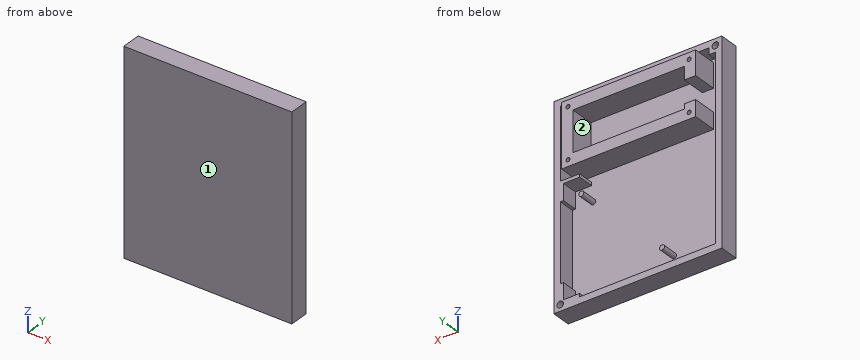
```python
from build123d import *

# Parameters (mm, degrees)
SKETCH1_W           = 104
SKETCH1_H           = 124
BOSS_EXTRUDE1_DEPTH = 2
SKETCH2_W           = 104
SKETCH2_H           = 124
SKETCH2_R           = 2
SKETCH2_R_2         = 1.55
BOSS_EXTRUDE2_DEPTH = 10
SKETCH3_R           = 1.25
BOSS_EXTRUDE3_DEPTH = 15


with BuildPart() as part:
    # Sketch1 → Boss-Extrude1 (new body)
    with BuildSketch(Plane(origin=(0, 0, 0), x_dir=(1, 0, 0), z_dir=(0, 1, 0))):
        Rectangle(SKETCH1_W, SKETCH1_H)
    extrude(amount=BOSS_EXTRUDE1_DEPTH)

    # Sketch2 → Boss-Extrude2 (add)
    # profile 1 of 3: a face of its own
    with BuildSketch(Plane(origin=(0, 2, 0), x_dir=(1, 0, 0), z_dir=(0, 1, 0))):
        Rectangle(SKETCH2_W, SKETCH2_H)
        Polygon((36, -14), (48, -14), (48, -58), (-44, -58), (-44, -54), (-48, -54), (-48, 58), (36, 58), (36, 56), (46, 56), (46, 46), (48, 46), (48, -2), (46, -2), (46, -12), (36, -12), align=None, mode=Mode.SUBTRACT)
        with Locations(Location((48, 58, 0), (0, 0, 270))):
            Circle(SKETCH2_R, mode=Mode.SUBTRACT)
        with Locations(Location((-48, -58, 0), (0, 0, 270))):
            Circle(SKETCH2_R, mode=Mode.SUBTRACT)
    # profile 2 of 3: a face of its own
    with BuildSketch(Plane(origin=(0, 2, 0), x_dir=(1, 0, 0), z_dir=(0, 1, 0))):
        with Locations(Location((-15, 48, 0), (0, 0, 90))):
            Circle(SKETCH2_R_2)
    # profile 3 of 3: a face of its own
    with BuildSketch(Plane(origin=(0, 2, 0), x_dir=(1, 0, 0), z_dir=(0, 1, 0))):
        with Locations(Location((35, -2, 0), (0, 0, 90))):
            Circle(SKETCH2_R_2)
    extrude(amount=BOSS_EXTRUDE2_DEPTH)

    # Sketch3 → Boss-Extrude3 (add)
    with BuildSketch(Plane(origin=(0, 2, 0), x_dir=(1, 0, 0), z_dir=(0, 1, 0))):
        Polygon((36.5, -49), (-32.5, -49), (-32.5, -41), (-39.5, -41), (-39.5, -56), (43.5, -56), (43.5, -17), (-39.5, -17), (-39.5, -27), (-32.5, -27), (-32.5, -24), (36.5, -24), align=None)
        with Locations(Location((-35.5, -52, 0), (0, 0, 270))):
            Circle(SKETCH3_R, mode=Mode.SUBTRACT)
        with Locations(Location((39.5, -52, 0), (0, 0, 270))):
            Circle(SKETCH3_R, mode=Mode.SUBTRACT)
        with Locations(Location((-35.5, -21, 0), (0, 0, 270))):
            Circle(SKETCH3_R, mode=Mode.SUBTRACT)
        with Locations(Location((39.5, -21, 0), (0, 0, 270))):
            Circle(SKETCH3_R, mode=Mode.SUBTRACT)
    extrude(amount=BOSS_EXTRUDE3_DEPTH)


solid = part.part
```
Can you work these out from the model? Positions are in its coordinate system, mm. Face numbers are marked on the shaded views. Round coordinates to 2 decimals unless told otherwise and drop trailing zeros. Loops run counter-clockwise (first coordinate to the right, second up) from the corner with the lowest first, then second, coordinate; pieces in that order, holes last.
Item 1: Suppose I cut it at B-B, the plane x = -24. Write out the boundary of the cut face in (y, z), then the cut area to 3 significant figures.
Item 2: Will these pins go through, and if not, where does the flat tip stop? pin 1 Ø1.2 at (x, z) = (39.5, 21.5) entering from +Y; pin 2 Ø2.5 at (x, z) = (35.5, 2.5) entering from +Y; pin 3 Ø2 at (x, z) = (-35.5, 21) entering from -Y.
Item 3: Suppose I cut it at C-C, the plane z = 7.5. Write out the boundary of the cut face in (x, y).
Item 4: If we mould it in two halves opening along Z, with no side actions, what happens to the marked faces 1 and 2? For each: +Z half, -Z half, draft (parallel to the pull), parting line (faces both ways), or undercut.
Item 5: Suppose I cut it at A-A, the plane y = 7. State how many separate pieces and enclosed holes the cut face has, then the cut area to 3 significant figures.
Item 6: Suppose I cut it at D-D, the plane z = -15. Write out the boundary of the cut face in (x, y), then the cut area to 3 significant figures.
Item 7: Please list where these lines run through material, in increasing order: L1, parallel to X at y = 4, z = 47.5; L2, parallel to Z at x = -38.5, y = 11.25; L3, parallel to X at y = 8, z = 21.
Reported:
1. outline: (0, -62) - (12, -62) - (12, -58) - (2, -58) - (2, 17) - (17, 17) - (17, 24) - (2, 24) - (2, 49) - (17, 49) - (17, 56) - (2, 56) - (2, 58) - (12, 58) - (12, 62) - (0, 62) - close
1. area: 538 mm2
2. pin 1: stops at y = 2
2. pin 2: stops at y = 12
2. pin 3: stops at y = 0
3. outline: (-52, 0) - (52, 0) - (52, 12) - (46, 12) - (46, 2) - (-48, 2) - (-48, 12) - (-52, 12) - close
4. face 1: draft
4. face 2: undercut
5. separate pieces: 4
5. enclosed holes: 7
5. area: 3,250 mm2
6. outline: (-52, 0) - (52, 0) - (52, 12) - (48, 12) - (48, 2) - (-48, 2) - (-48, 12) - (-52, 12) - close
6. area: 288 mm2
7. L1: x = -52 to -48, -39.5 to -32.5, 36.5 to 43.5, 48 to 52
7. L2: z = -62 to -58, 17 to 27, 41 to 56, 58 to 62
7. L3: x = -52 to -48, -39.5 to -36.75, -34.25 to 38.25, 40.75 to 43.5, 48 to 52
